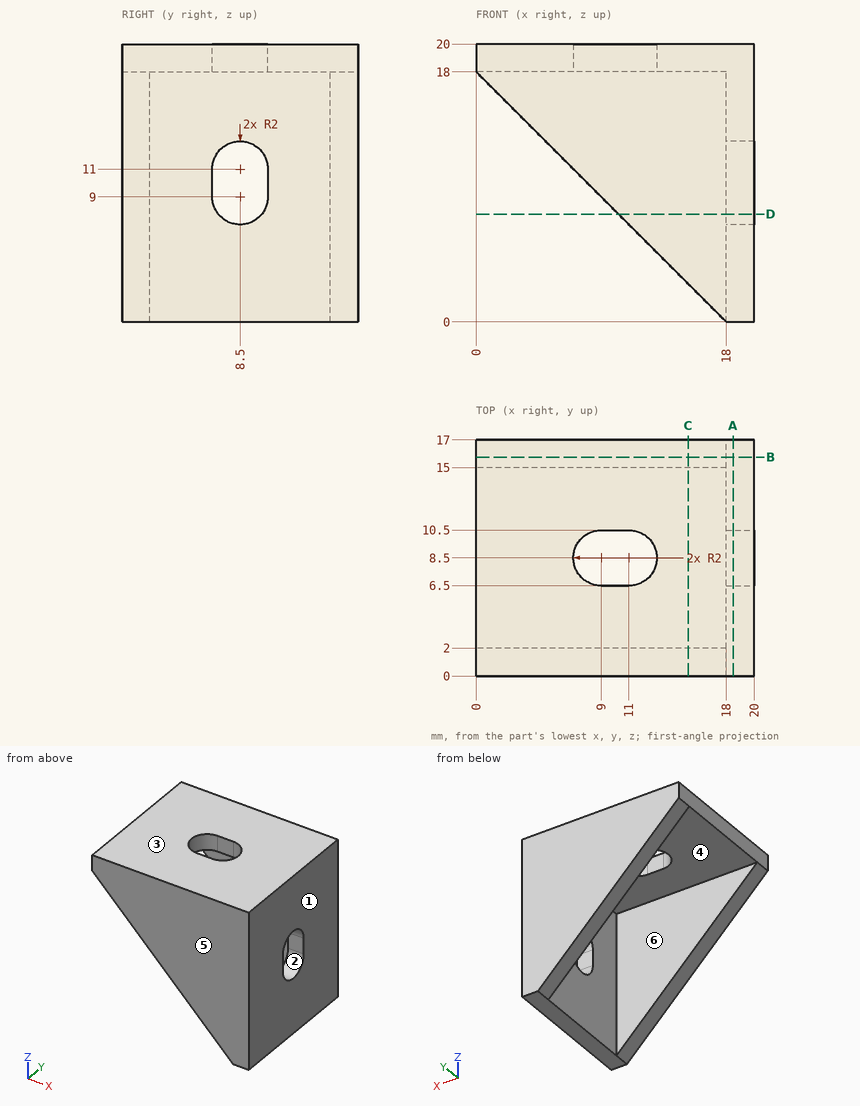
Verification items for this drawing (mm, ordinates from the low corner). A direction names the side the tool comes from. Coordinates: 2 decimals unless noted, no trailing zeros. Loops run counter-clockwise (first coordinate to the right, second up) from the corner with the lowest first, then second, coordinate; pieces in that order, holes last. Notation, with made-up numbers: (11, 77) -> (56, 77) arc R24 cw to (56, 103) -> close; hole circle Ø10 at (58, 25.25). An arc over 180 degrees is marked (long way). Answer in a Markdown table with one row per item. Add a question column.
1. Section check B-B, the plane y = 15.75. Enter the section's corners in (x, z).
2. Material ranges on probe 1 along Y at (x, z) = (13.5, 5); probe 2 along X at (y, z) = (9.5, 3.75), recorded low to high. Write a range as [from, to].
3. Depth check by flat-ended pin: P1, Ø1.5, axis at y = 9.5, z = 15, coming from the -X side. Enter the tip coordinate at first touch or a pass-through.
4. Section check D-D, the plane z = 7.75. Enter the section's corners in (x, y), then the cut area to 3 significant figures.
5. Section check A-A, the plane x = 18.5. Enter the section's corners in (y, z), then the cut area to 3 significant figures.
6. Draft check along Z on the marked faces 1, 2, 3 and 4. Enter one of: +Z half, -Z half, draft (parallel to the pull), parting line (faces both ways), or undercut.
7. Access from +Z, -Z, +X, -X, +Y, -Y to the whole of each face (thin tool, end or side, straight path). Record for the marked faces 5 and 6.
8. Section check C-C, the plane x = 15.25. Enter the section's corners in (y, z).
Derived:
| question | item | result |
|---|---|---|
| 1 | outline | (0, 18) -> (18, 0) -> (20, 0) -> (20, 20) -> (0, 20) -> close |
| 2 | probe 1 | y = [0, 2], [15, 17] |
| 2 | probe 2 | x = [18, 20] |
| 3 | P1 | stops at x = 18 |
| 4 | outline | (10.25, 0) -> (20, 0) -> (20, 6.94) -> (18, 6.94) -> (18, 2) -> (10.25, 2) -> close; (10.25, 15) -> (18, 15) -> (18, 10.06) -> (20, 10.06) -> (20, 17) -> (10.25, 17) -> close |
| 4 | area | 58.8 mm² |
| 5 | outline | (0, 0) -> (17, 0) -> (17, 20) -> (0, 20) -> close; hole (6.5, 9) arc R2 ccw to (10.5, 9) -> (10.5, 11) arc R2 ccw to (6.5, 11) -> close |
| 5 | area | 319 mm² |
| 6 | face 1 | draft |
| 6 | face 2 | undercut |
| 6 | face 3 | +Z half |
| 6 | face 4 | -Z half |
| 7 | face 5 | +Z, -Z, +X, -X, -Y |
| 7 | face 6 | -Z, -X |
| 8 | outline | (0, 2.75) -> (2, 2.75) -> (2, 18) -> (15, 18) -> (15, 2.75) -> (17, 2.75) -> (17, 20) -> (0, 20) -> close |
